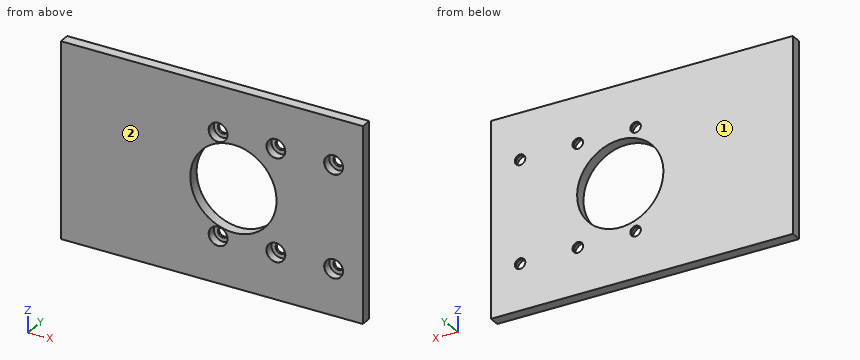
from build123d import *

# Parameters (mm, degrees)
SKETCH1_W                       = 88.9
SKETCH1_H                       = 57.15
BOSS_EXTRUDE1_DEPTH             = 1.5875
SKETCH2_R                       = 12.7
CUT_EXTRUDE1_DEPTH              = 3.175
CBORE_FOR_M2_5_SHCS1_AT_2_COUNT = 2
CBORE_FOR_M2_5_SHCS1_AT_2_PITCH = 17
CBORE_FOR_M2_5_SHCS1_AT_3_COUNT = 2
CBORE_FOR_M2_5_SHCS1_AT_3_PITCH = 34
CBORE_FOR_M2_5_SHCS1_AT_4_COUNT = 2
CBORE_FOR_M2_5_SHCS1_AT_4_PITCH = 30
CBORE_FOR_M2_5_SHCS1_AT_5_COUNT = 2
CBORE_FOR_M2_5_SHCS1_AT_5_PITCH = 34.481879299
CBORE_FOR_M2_5_SHCS1_AT_6_COUNT = 2
CBORE_FOR_M2_5_SHCS1_AT_6_PITCH = 45.343136195


with BuildPart() as part:
    # Sketch1 → Boss-Extrude1 (new, symmetric)
    with BuildSketch(Plane(origin=(0, 0, 0), x_dir=(1, 0, 0), z_dir=(0, 1, 0))):
        with Locations((-6.35, 0)):
            Rectangle(SKETCH1_W, SKETCH1_H)
    extrude(amount=BOSS_EXTRUDE1_DEPTH, both=True)

    # Sketch2 → Cut-Extrude1 (cut)
    with BuildSketch(Plane(origin=(0, 1.5875, 0), x_dir=(1, 0, 0), z_dir=(0, 1, 0))):
        with Locations(Location((0, 0, 0), (0, 0, 270))):
            Circle(SKETCH2_R)
    extrude(amount=-CUT_EXTRUDE1_DEPTH, mode=Mode.SUBTRACT)

    # Sketch10 → CBORE for M2.5 SHCS1 (revolve, cut)
    with BuildSketch(Plane(origin=(29.5, -1.5875, -15), x_dir=(0, 0, -1), z_dir=(1, 0, 0))):
        Polygon((0, 0), (0, 153.331333959), (1.55, 152.4), (1.55, 2.5), (2.75, 2.5), (2.75, 0.025), (2.775, 0), align=None)
    cbore_for_m2_5_shcs1 = revolve(axis=Axis((29.5, -7.9375, -15), (0, 1, 0)), mode=Mode.SUBTRACT)

    # CBORE for M2.5 SHCS1 at 2: CBORE for M2.5 SHCS1 ×2
    with Locations(*[(-i * CBORE_FOR_M2_5_SHCS1_AT_2_PITCH, 0, 0) for i in range(1, CBORE_FOR_M2_5_SHCS1_AT_2_COUNT)]):
        add(cbore_for_m2_5_shcs1, mode=Mode.SUBTRACT)

    # CBORE for M2.5 SHCS1 at 3: CBORE for M2.5 SHCS1 ×2
    with Locations(*[(-i * CBORE_FOR_M2_5_SHCS1_AT_3_PITCH, 0, 0) for i in range(1, CBORE_FOR_M2_5_SHCS1_AT_3_COUNT)]):
        add(cbore_for_m2_5_shcs1, mode=Mode.SUBTRACT)

    # CBORE for M2.5 SHCS1 at 4: CBORE for M2.5 SHCS1 ×2
    with Locations(*[(0, 0, i * CBORE_FOR_M2_5_SHCS1_AT_4_PITCH) for i in range(1, CBORE_FOR_M2_5_SHCS1_AT_4_COUNT)]):
        add(cbore_for_m2_5_shcs1, mode=Mode.SUBTRACT)

    # CBORE for M2.5 SHCS1 at 5: CBORE for M2.5 SHCS1 ×2
    with Locations(*[Vector(-0.49301257198088044, 0, 0.8700221858486122) * (i * CBORE_FOR_M2_5_SHCS1_AT_5_PITCH) for i in range(1, CBORE_FOR_M2_5_SHCS1_AT_5_COUNT)]):
        add(cbore_for_m2_5_shcs1, mode=Mode.SUBTRACT)

    # CBORE for M2.5 SHCS1 at 6: CBORE for M2.5 SHCS1 ×2
    with Locations(*[Vector(-0.7498378553650926, 0, 0.6616216370868463) * (i * CBORE_FOR_M2_5_SHCS1_AT_6_PITCH) for i in range(1, CBORE_FOR_M2_5_SHCS1_AT_6_COUNT)]):
        add(cbore_for_m2_5_shcs1, mode=Mode.SUBTRACT)


solid = part.part
Input: part model. Units: mm. Frame: model coordinates. Face numbers are marked on the shaded views. Coordinates: 2 decimals unless noted, no trailing zeros. Loops run counter-clockwise (first coordinate to the right, second up) from the corner with the lowest first, then second, coordinate; pieces in that order, holes last. Notation, with made-up numbers: (83.25, 9.25) - (126.25, 9.25) arc R17 ccw to (126.25, 20.25) - close; hole circle Ø10 at (8, 57). An arc over 180 degrees is marked (long way). Answer in a Markdown table with one row per item. Add a question column.
Item 1: Contact query for flat-ended pins moving along their axis: P1, Ø4, axis at x = 29.5, z = 15, coming from the -Y side; P2, Ø1.6, axis at x = 12.5, z = 14.5, coming from the -Y side. Output: stop coordinate, or through.
Item 2: Section query D-D on x = 0. Return the cut outline in (y, z) (1 decimal).
Item 3: Line query: line 1 along X through (y, z) = (0.75, -17); line 2 along X through (y, z) = (-0.65, 4); line 3 along X through (y, z) = (-0.15, -14). Output: solid intervals per line, ascending. Write a range as [from, to].
Item 4: Section query B-B on y = 0.15. Return the cut outline in (x, z) (3 decimals).
Item 5: Mould query, pull axis Y, two halves, no side actions, for the marked faces 1 and 2. Classes: released by +Y, released by -Y, zero draft, split by the parting line, or undercut.
Item 6: Section query C-C on z = 15. State how many separate pieces and enclosed holes the cut face has, then the cut area to 3 significant figures.
Item 7: Section query A-A on z = 0. Return the cut outline in (x, y), then the cut area to 3 significant figures.
Recorded:
| question | item | result |
|---|---|---|
| 1 | P1 | y = 0.91 |
| 1 | P2 | through |
| 2 | outline | (-1.6, -28.6) - (1.6, -28.6) - (1.6, -12.7) - (-1.6, -12.7) - close; (-1.6, 12.7) - (1.6, 12.7) - (1.6, 28.6) - (-1.6, 28.6) - close |
| 3 | line 1 | [-50.8, -6.39], [-2.61, 10.61], [14.39, 27.61], [31.39, 38.1] |
| 3 | line 2 | [-50.8, -12.05], [12.05, 38.1] |
| 3 | line 3 | [-50.8, -7.06], [-1.94, 9.94], [15.06, 26.94], [32.06, 38.1] |
| 4 | outline | (-50.8, -28.575) - (38.1, -28.575) - (38.1, 28.575) - (-50.8, 28.575) - close; hole circle Ø25.4 at (0, 0); hole circle Ø5.5 at (-4.5, -15); hole circle Ø5.5 at (-4.5, 15); hole circle Ø5.5 at (12.5, -15); hole circle Ø5.5 at (12.5, 15); hole circle Ø5.5 at (29.5, -15); hole circle Ø5.5 at (29.5, 15) |
| 5 | face 1 | released by +Y |
| 5 | face 2 | released by -Y |
| 6 | separate pieces | 4 |
| 6 | enclosed holes | 0 |
| 6 | area | 235 mm^2 |
| 7 | outline | (-50.8, -1.59) - (-12.7, -1.59) - (-12.7, 1.59) - (-50.8, 1.59) - close; (12.7, -1.59) - (38.1, -1.59) - (38.1, 1.59) - (12.7, 1.59) - close |
| 7 | area | 202 mm^2 |
